from build123d import *

# Parameters (mm, degrees)
F0_R     = 1.5
F1_DEPTH = 1.6


with BuildPart() as f1:
    # F0 (on Top) → F1 (new body)
    with BuildSketch(Plane.XY):
        Polygon((210, 8.27), (210, 106.65), (0, 106.65), (0, 0), (15, 0), (15, 8.25), (29.7, 8.25), (29.7, 0), (41.35, 0), (41.35, 8.25), (45, 8.25), (45, -4.5), (56.2, -4.5), (56.2, 8.27), (58.1, 8.27), (58.1, -4.5), (96.3, -4.5), (96.3, 8.27), align=None)
        with Locations((7.5, 4.87)):
            Circle(F0_R, mode=Mode.SUBTRACT)
    extrude(amount=F1_DEPTH)


solid = f1.part
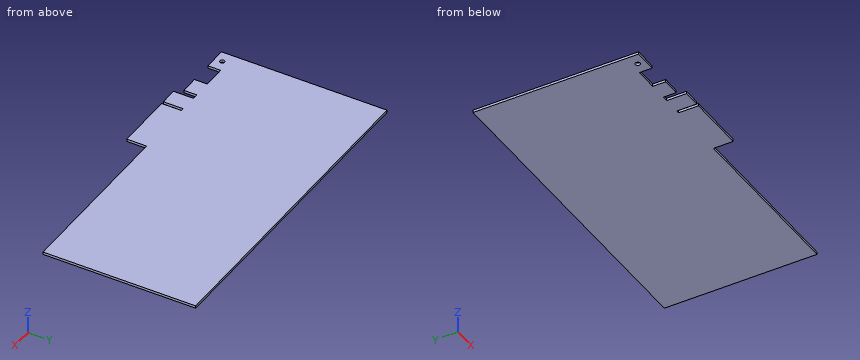
Can you work these out from the model? Positions are in its coordinate system, mm. Coordinates: 2 decimals unless noted, no trailing zeros. Write each loop counter-clockwise with the first axis right and the second up, starting at its lowest first coordinate (ties: lowest second). Pieces come first, ordered by that corner, then holes. Notation, with made-up numbers: (68.25, 86.5) -> (94.25, 86.5) arc R25 ccw to (94.25, 117.5) -> close; hole circle Ø3 at (9, 45). An arc over 180 degrees is marked (long way). Write each question's results on one line, items separated by ' | '. Start each with the question number.
Item 1: If we section it at A-A, the plane z = 0.3: Write out the boundary of the cut face in (x, y), and give its area (3 significant figures).
Item 2: Please list where these lines run through material, in increasing order: probe 1 along Y at (x, z) = (7.5, 0.9); probe 2 along Y at (x, z) = (10.5, 0.6); probe 3 along Y at (x, z) = (128.5, 1.1).
Item 3: If we section it at B-B, the plane x = 127: Write out the boundary of the cut face in (y, z), and give its area (3 significant figures).
Item 4: I'm going to push flat-ended pins straight in: P1, Ø0.5, axis at x = 43, z = 0.5, coming from the -Y side; P2, Ø1.8, axis at x = 7.5, y = 4.87, coming from the -Z side; P3, Ø0.8, axis at y = 0.5, z = 1, coming from the +X side; P4, Ø0.5, axis at x = 57.5, z = 1, coming from the -Y side. Where does each tip first touch, or does it pass through?
Answer block:
1) outline: (0, 0) -> (15, 0) -> (15, 8.25) -> (29.7, 8.25) -> (29.7, 0) -> (41.35, 0) -> (41.35, 8.25) -> (45, 8.25) -> (45, -4.5) -> (56.2, -4.5) -> (56.2, 8.27) -> (58.1, 8.27) -> (58.1, -4.5) -> (96.3, -4.5) -> (96.3, 8.27) -> (210, 8.27) -> (210, 106.65) -> (0, 106.65) -> close; hole circle Ø3 at (7.5, 4.87) | area: 21,500 mm²
2) probe 1: 0 to 3.37, 6.37 to 106.65 | probe 2: 0 to 106.65 | probe 3: 8.27 to 106.65
3) outline: (8.27, 0) -> (106.65, 0) -> (106.65, 1.6) -> (8.27, 1.6) -> close | area: 157 mm²
4) P1: y = 8.25 | P2: through | P3: x = 96.3 | P4: y = 8.27
